Geometry: final body of the model. Coordinates: model frame, mm. A direction names the side the tool comes from. Round coordinates to 2 decimals unless told otherwise and drop trailing zeros. Order: outer loops, then holes, each group sorted by start corner. A loop starts at its lowest first (then second) coordinate and runs counter-clockwise, first axis right, second up. Notation, with made-up numbers: (-24, 22.25) -> (-8, 22.25) arc R17 ccw to (-8, 34.25) -> close; hole circle Ø5 at (2, 8.25). An arc over 180 degrees is marked (long way). Put each result on its own line as item: value.
```python
from build123d import *

# Parameters (mm, degrees)
SKETCH1_W           = 240
SKETCH1_H           = 351.15
BOSS_EXTRUDE3_DEPTH = 21
SKETCH5_W           = 248.975913499
SKETCH5_H           = 113.170869772
CUT_EXTRUDE5_DEPTH  = 254
CAVITY1_START       = -93.176553254
CAVITY1_DEPTH       = 230
SKETCH6_W           = 230
SKETCH6_H           = 2.384694545
CUT_EXTRUDE6_DEPTH  = 10
SKETCH7_W           = 329.692379319
SKETCH7_H           = 158.801284786
CUT_EXTRUDE8_DEPTH  = 33
CUT_EXTRUDE9_DEPTH  = 10


with BuildPart() as part:
    # Sketch1 → Boss-Extrude3 (new body)
    with BuildSketch(Plane(origin=(0, 0, 0), x_dir=(1, 0, 0), z_dir=(0, 1, 0))):
        with Locations((21.823446746, 98.176553254)):
            Rectangle(SKETCH1_W, SKETCH1_H)
    extrude(amount=BOSS_EXTRUDE3_DEPTH)

    # Sketch5 → Cut-Extrude5 (cut)
    with BuildSketch(Plane(origin=(0, 0, -54.481553254), x_dir=(-1, 0, 0), z_dir=(0, 0, -1))):
        with Locations((-20.8478358, 4.110963623)):
            Rectangle(SKETCH5_W, SKETCH5_H)
    extrude(amount=CUT_EXTRUDE5_DEPTH, mode=Mode.SUBTRACT)

    # Cavity1: read off the stored shape, not the designer's step
    # Cavity1 outline → Cavity1 (cut)
    with BuildSketch(Plane.YZ.offset(CAVITY1_START)):
        Polygon((18.5, 60.403141291), (13.5, 67.518446746), (13.5, 67.903141291), (18.5, 67.903141291), (13.5, 75.018446746), (5, 75.018446746), (5, -54.481553254), (13.5, -54.481553254), (13.5, -52.096858709), (18.5, -52.096858709), (13.5, -44.981553254), (13.5, -44.596858709), (18.5, -44.596858709), (13.5, -37.481553254), (13.5, -37.096858709), (18.5, -37.096858709), (13.5, -29.981553254), (13.5, -29.596858709), (18.5, -29.596858709), (13.5, -22.481553254), (13.5, -22.096858709), (18.5, -22.096858709), (13.5, -14.981553254), (13.5, -14.596858709), (18.5, -14.596858709), (13.5, -7.481553254), (13.5, -7.096858709), (18.5, -7.096858709), (13.5, 0.018446746), (13.5, 0.403141291), (18.5, 0.403141291), (13.5, 7.518446746), (13.5, 7.903141291), (18.5, 7.903141291), (13.5, 15.018446746), (13.5, 15.403141291), (18.5, 15.403141291), (13.5, 22.518446746), (13.5, 22.903141291), (18.5, 22.903141291), (13.5, 30.018446746), (13.5, 30.403141291), (18.5, 30.403141291), (13.5, 37.518446746), (13.5, 37.903141291), (18.5, 37.903141291), (13.5, 45.018446746), (13.5, 45.403141291), (18.5, 45.403141291), (13.5, 52.518446746), (13.5, 52.903141291), (18.5, 52.903141291), (13.5, 60.018446746), (13.5, 60.403141291), align=None)
    extrude(amount=CAVITY1_DEPTH, mode=Mode.SUBTRACT)

    # Sketch6 → Cut-Extrude6 (cut)
    with BuildSketch(Plane(origin=(0, 13.5, 0), x_dir=(-1, 0, 0), z_dir=(0, -1, 0))):
        with Locations((-21.823446746, 53.289205982)):
            Rectangle(SKETCH6_W, SKETCH6_H)
    extrude(amount=-CUT_EXTRUDE6_DEPTH, mode=Mode.SUBTRACT)

    # Sketch7 → Cut-Extrude8 (cut)
    with BuildSketch(Plane(origin=(0, 13.5, 0), x_dir=(-1, 0, 0), z_dir=(0, -1, 0))):
        with Locations((-33.84938791, -12.885366014)):
            Rectangle(SKETCH7_W, SKETCH7_H)
    extrude(amount=-CUT_EXTRUDE8_DEPTH, mode=Mode.SUBTRACT)

    # Sketch9 → Cut-Extrude9 (cut)
    with BuildSketch(Plane(origin=(0, 13.5, 0), x_dir=(1, 0, 0), z_dir=(0, 1, 0))):
        Polygon((139.223446746, 54.481553254), (139.223446746, -75.718446746), (-95.576553254, -75.718446746), (-95.576553254, 54.481553254), (-98.176553254, 54.481553254), (-98.176553254, -77.398446746), (141.823446746, -77.398446746), (141.823446746, 54.481553254), align=None)
    extrude(amount=-CUT_EXTRUDE9_DEPTH, mode=Mode.SUBTRACT)


solid = part.part
```
1. Set-up query: faces 1 (the face through (-95.577, 9, 12)), 2 (the face through (20, 9, 75.018)), 3 (the face through (23, 9, 75.718)). Return all of +Z, -Z, +X, -X, +Y, -Y with unobstructed straight access to the full face (end or side cutting, diameter ignored); none if empty.
Ans:
face 1: +Z, -Z, -X, +Y
face 2: -Z, +Y
face 3: +Z, +X, -X, +Y
2. Cut plane B-B on y = 10. Return loops of the section in (x, z).
Ans:
outline: (-95.58, -54.48) -> (-93.18, -54.48) -> (-93.18, 75.02) -> (136.82, 75.02) -> (136.82, -54.48) -> (139.22, -54.48) -> (139.22, 75.72) -> (-95.58, 75.72) -> close
3. Cut plane C-C on x = 33. Return loops of the section in (y, z), and give its area (3 significant figures).
Ans:
outline: (0, -54.48) -> (5, -54.48) -> (5, 75.02) -> (13.5, 75.02) -> (13.5, 75.72) -> (3.5, 75.72) -> (3.5, 77.4) -> (0, 77.4) -> close
area: 663 mm²
4. Contact query for flat-ended pins moving along their axis: P1, Ø7, axis at y = 9.5, z = -13.5, coming from the -X side; P2, Ø1, axis at x = -16.5, y = 10.5, coming from the +Z side; P3, Ø7, axis at x = -4.5, y = 11.5, coming from the -Z side. Output: stop coordinate, or through.
Ans:
P1: x = -95.58
P2: z = 75.72
P3: z = 75.02
5. Material intervals for probe 1 along X at (y, z) = (7.25, 48); probe 2 along Y at (x, z) = (57, 1); probe 3 along X at (y, z) = (4, -45.5), sorted ascending.
Ans:
probe 1: -95.58 to -93.18, 136.82 to 139.22
probe 2: 0 to 5
probe 3: -95.58 to 139.22
6. Draft query along X for faces 4 (the face through (20, 0, 11)), 5 (the face through (139.223, 9, 10)), 6 (the face through (20, 5, 11)). Return one class per face: +X half, -X half, draft (parallel to the pull), parting line (faces both ways), or undercut.
Ans:
face 4: draft
face 5: +X half
face 6: undercut
7. Cut plane A-A on z = 23.5. Return loops of the section in (x, y), and give its area (3 significant figures).
Ans:
outline: (-98.18, 0) -> (141.82, 0) -> (141.82, 3.5) -> (139.22, 3.5) -> (139.22, 13.5) -> (136.82, 13.5) -> (136.82, 5) -> (-93.18, 5) -> (-93.18, 13.5) -> (-95.58, 13.5) -> (-95.58, 3.5) -> (-98.18, 3.5) -> close
area: 1,230 mm²
